```python
from build123d import *

# Parameters (mm, degrees)
EXTRUDE_1_DEPTH            = 6.5
HOLE_WIZARD_M81_AT_2_COUNT = 2
HOLE_WIZARD_M81_AT_2_PITCH = 18
CHAMFER_1_SIZE             = 0.5


with BuildPart() as part:
    # Эскиз1 → Бобышка-Вытянуть1 (new body, symmetric)
    with BuildSketch(Plane.XY):
        with BuildLine():
            Line((0, 50), (0, 7))
            ThreePointArc((0, 7), (2.050252532, 2.050252532), (7, 0))
            Line((7, 0), (50, 0))
            Line((50, 0), (50, 5.5))
            Line((50, 5.5), (7, 5.5))
            ThreePointArc((7, 5.5), (5.939339828, 5.939339828), (5.5, 7))
            Line((5.5, 7), (5.5, 50))
            Line((5.5, 50), (0, 50))
        make_face()
    extrude(amount=EXTRUDE_1_DEPTH, both=True)

    # Эскиз5 → Отверстие обработанное метчиком M81 (revolve, cut)
    with BuildSketch(Plane.ZX.offset(35)):
        Polygon((0, 0), (0, 5.5), (4.2, 5.5), (3.4, 4.7), (3.4, 0.8), (4.2, 0), align=None)
    hole_wizard_m81 = revolve(axis=Axis((-6.35, 35, 0), (1, 0, 0)), mode=Mode.SUBTRACT)

    # Отверстие обработанное метчиком M81 at 2: Отверстие обработанное метчиком M81 ×2
    with Locations(*[(0, -i * HOLE_WIZARD_M81_AT_2_PITCH, 0) for i in range(1, HOLE_WIZARD_M81_AT_2_COUNT)]):
        add(hole_wizard_m81, mode=Mode.SUBTRACT)

    # Зеркальное отражение1: Отверстие обработанное метчиком M81 across plane
    add(hole_wizard_m81.mirror(Plane(origin=(0, 0, 0), x_dir=(0, 0, 1), z_dir=(-0.707106781, 0.707106781, 0))), mode=Mode.SUBTRACT)

    # Зеркальное отражение1 copy 1 sketch → Зеркальное отражение1 copy 1 (revolve, cut)
    with BuildSketch(Plane(origin=(17, 0, 0), x_dir=(0, 0, 1), z_dir=(1, 0, 0))):
        Polygon((0, 0), (0, -5.5), (4.2, -5.5), (3.4, -4.7), (3.4, -0.8), (4.2, 0), align=None)
    revolve(axis=Axis((17, -6.35, 0), (0, -1, 0)), mode=Mode.SUBTRACT)

    # Фаска1
    chamfer_1_edges = [part.edges().sort_by_distance(p)[0] for p in [
        (2.75, 50, -6.5),
        (50, 2.75, 6.5),
        (2.75, 50, 6.5),
        (50, 2.75, -6.5),
    ]]
    chamfer(chamfer_1_edges, length=CHAMFER_1_SIZE)


solid = part.part
```
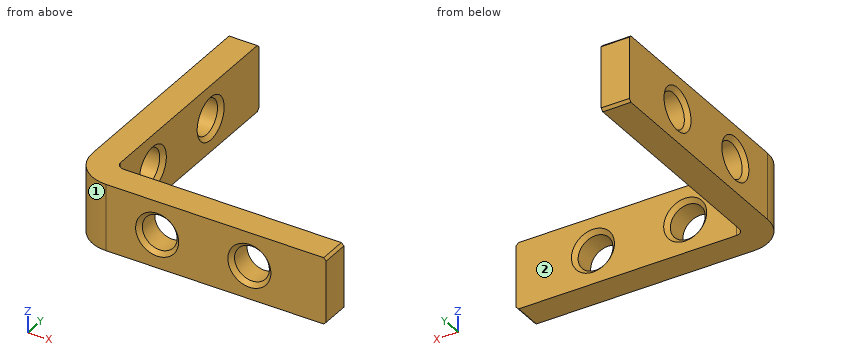
The model under review builds one solid part; all positions refer to its coordinate system, in mm. Face numbers are marked on the shaded views. A direction names the side the tool comes from. Round coordinates to 2 decimals unless told otherwise and drop trailing zeros. Loops run counter-clockwise (first coordinate to the right, second up) from the corner with the lowest first, then second, coordinate; pieces in that order, holes last.
Item 1: Take a section at D-D (z = 0). Give the number of separate pieces and of enclosed holes in the cut face, then the cut area to 3 significant figures.
Determined:
separate pieces: 5
enclosed holes: 0
area: 355 mm2
Item 2: Take a section at C-C (z = 5). Write out the cut boundary in (x, y), then the cut area to 3 significant figures.
Determined:
outline: (0, 7) arc R7 ccw to (7, 0) - (50, 0) - (50, 5.5) - (7, 5.5) arc R1.5 cw to (5.5, 7) - (5.5, 50) - (0, 50) - close
area: 510 mm2
Item 3: For the marked faces 1 and 2, list the 3-axis set-ups (+Z, -Z, +X, -X, +Y, -Y) from which the entire face can be reached by the end or side of a thin tool; tool diameter is ignored.
Determined:
face 1: +Z, -Z, -X, -Y
face 2: +Z, -Z, +X, +Y
Item 4: Clearance check with flat-ended pins moving along their axes: pin 1 Ø4 at (x, z) = (15.5, 0) entering from -Y; pin 2 Ø5.5 at (x, z) = (17, 0) entering from -Y; pin 3 Ø3 at (x, z) = (37.5, 0.5) entering from +Y; pin 4 Ø2 at (y, z) = (40.5, 5) entering from +X. State where each tip first meets the part, or that it passes through.
Determined:
pin 1: stops at y = 0.7
pin 2: passes through
pin 3: stops at y = 5.35
pin 4: stops at x = 5.5
Item 5: For line 1 (Z direction, x = 2, y = 35); line 2 (X direction, y = 3.1, z = 0); line 3 (X direction, y = 2.5, z = 0), list the stretches that pass through material, from the lowest coordinate up.
Determined:
line 1: z = -6.5 to -3.4, 3.4 to 6.5
line 2: x = 1.19 to 13.6, 20.4 to 31.6, 38.4 to 50
line 3: x = 1.64 to 13.6, 20.4 to 31.6, 38.4 to 50
Item 6: Take a section at A-A (x = 17). Write out the cut boundary in (y, z), then the cut area to 3 significant figures.
Determined:
outline: (0, -6.5) - (5.5, -6.5) - (5.5, -4.2) - (4.7, -3.4) - (0.8, -3.4) - (0, -4.2) - close; (0, 4.2) - (0.8, 3.4) - (4.7, 3.4) - (5.5, 4.2) - (5.5, 6.5) - (0, 6.5) - close
area: 32.8 mm2
